Autodesk Inventor part; units mm, degrees
ref_plane "YZ Plane" through (0, 0, 0) normal (1, 0, 0) x (0, 1, 0)
ref_plane "XZ Plane" through (0, 0, 0) normal (0, 1, 0) x (-1, 0, 0)
ref_plane "XY Plane" through (0, 0, 0) normal (0, 0, 1) x (1, 0, 0)
sketch "Sketch1" plane through (0, 0, 0) normal (1, 0, 0) x (0, 1, 0)
  circle A0 centre (0, 0) radius 12.7
  circle A1 centre (0, 0) radius 111.9
  dimension "D_eje" = 25.4
  dimension "d1" = 223.8
extrude "Extrusion1" add sketch "Sketch1" along normal blind 9
sketch "Sketch2" plane through (9, 0, 0) normal (1, 0, 0) x (0, 0, -1)
  line L0 (6, 19.0264) -> (6, 99.7197)
  line L1 (0, -188.1875) -> (0, 173.8632) construction
  arc A0 (0, 19.95) -> (-13.4773, 14.7093) centre (0, 0) ccw construction
  circle A1 centre (0, 0) radius 12.7 construction
  arc A2 (0, 99.9) -> (86.5159, -49.95) centre (0, 0) ccw construction
  line L2 (181.1282, 0) -> (-189.3983, 0) construction
  arc A3 (6, 19.0264) -> (0, 19.95) centre (0, 0) ccw construction
  arc A4 (-19.95, 0) -> (0, -19.95) centre (0, 0) ccw construction
  arc A5 (0, -19.95) -> (17.2772, -9.975) centre (0, 0) ccw construction
  arc A6 (19.95, 0) -> (6, 19.0264) centre (0, 0) ccw
  line L3 (0, 0) -> (86.5159, -49.95) construction
  line L4 (19.4773, -4.317) -> (89.3598, -44.6637)
  arc A7 (-13.4773, 14.7093) -> (-19.95, 0) centre (0, 0) ccw construction
  arc A8 (19.4773, -4.317) -> (19.95, 0) centre (0, 0) ccw
  arc A9 (17.2772, -9.975) -> (19.4773, -4.317) centre (0, 0) ccw construction
  arc A10 (6, 99.7197) -> (0, 99.9) centre (0, 0) ccw construction
  arc A11 (86.5159, -49.95) -> (89.3598, -44.6637) centre (0, 0) ccw construction
  arc A12 (89.3598, -44.6637) -> (6, 99.7197) centre (0, 0) ccw
  line L5 (-19.4773, -4.317) -> (-89.3598, -44.6637)
  arc A13 (-6, 99.7197) -> (-89.3598, -44.6637) centre (0, 0) ccw
  line L6 (-6, 19.0264) -> (-6, 99.7197)
  arc A14 (-9.975, 17.2772) -> (-19.4773, -4.317) centre (0, 0) ccw
  line L7 (13.4773, -14.7093) -> (83.3598, -55.056)
  arc A15 (-83.3598, -55.056) -> (83.3598, -55.056) centre (0, 0) ccw
  line L8 (-13.4773, -14.7093) -> (-83.3598, -55.056)
  arc A16 (-9.975, -17.2772) -> (13.4773, -14.7093) centre (0, 0) ccw
  point P0 (-6, -19.0264)
  point P1 (19.4773, 4.317)
  dimension "d4" = 6
  dimension "d7" = 39.9
  dimension "d8" = 199.8
  dimension "d10" = 120
  dimension "d11" = 6
  dimension "d14" = 360
extrude "Extrusion2" cut sketch "Sketch2" against normal blind 9
pattern_circular "Circular Pattern1" count 3 over 360 about axis through (-10, 0, 0) along (1, 0, 0) of "Extrusion2"
fillet "Fillet1" radius 2 12 edges at (4.5, -14.7093, -13.4773) (4.5, -14.7093, 13.4773) (4.5, -55.056, 83.3598) (4.5, -55.056, -83.3598) (4.5, -44.6637, -89.3598) (4.5, 99.7197, -6) (4.5, -4.317, -19.4773) (4.5, 19.0264, -6) (4.5, 19.0264, 6) (4.5, -4.317, 19.4773) (4.5, 99.7197, 6) (4.5, -44.6637, 89.3598)
properties part number "Rueda_triciclo" material "Aluminum 6061"
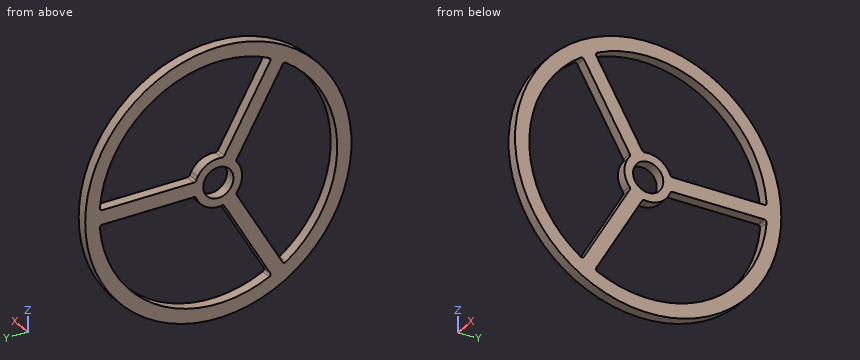
CAD build for the part. Positions are in the model's coordinates, mm. Give positions to 0.01 mm unless a question says otherwise; leave off trailing zeros. Order: outer loops, then holes, each group sorted by start corner. A loop starts at its lowest first (then second) coordinate and runs counter-clockwise, first axis right, second up.
(1) Saw through at C-C, the plane y = 68.5. Give the cut face in (x, z), then the cut area to 3 significant figures.
(2) Saw through at D-D, the plane x = 3.25. State how many separate pieces and enclosed holes the cut face has, then the cut area to 3 significant figures.
(3) Saw through at A-A, the plane z = 0. Give the cut face in (x, y), then the cut area to 3 significant figures.
(4) Drill centre lines: L1, parallel to Z at x = 2, y = 0; L2, parallel to Z at x = 1.5, y = 26.5; L3, parallel to Z at x = 5.75, y = -5.5. Where is each one in solid material? Low to high.
(5) Saw through at B-B, the plane y = -24.5. Give the cut face in (x, z).
(6) Flat gauge pins, fed straight in: pin 1 (1.5 mm diameter, centred on x = 6, z = 69.5, fed in from +Y); pin 2 (2 mm diameter, centred on x = 2.5, y = -34.5, fed in from -Z); pin 3 (4.5 mm diameter, centred on x = 4.5, y = 40.5, fed in from +Z); pin 4 (4 mm diameter, centred on y = 46, z = 88, fed in from -X). Where does each tip first touch, or does it go through?
Results found:
1. outline: (0, -88.48) - (9, -88.48) - (9, -72.72) - (0, -72.72) - close; (0, -6) - (9, -6) - (9, 6) - (0, 6) - close; (0, 72.72) - (9, 72.72) - (9, 88.48) - (0, 88.48) - close
1. area: 392 mm2
2. separate pieces: 1
2. enclosed holes: 4
2. area: 11,600 mm2
3. outline: (0, -111.9) - (9, -111.9) - (9, -99.9) - (0, -99.9) - close; (0, -19.95) - (9, -19.95) - (9, -12.7) - (0, -12.7) - close; (0, 12.7) - (9, 12.7) - (9, 111.9) - (0, 111.9) - close
3. area: 1,070 mm2
4. L1: z = -111.9 to -99.9, -19.95 to -12.7, 12.7 to 19.95, 99.9 to 111.9
4. L2: z = -108.72 to -96.32, -6 to 6, 96.32 to 108.72
4. L3: z = -111.76 to -99.75, -21.53 to -11.45, 11.45 to 21.53, 99.75 to 111.76
5. outline: (0, -109.18) - (9, -109.18) - (9, -96.85) - (0, -96.85) - close; (0, -54.44) - (9, -54.44) - (9, -30.44) - (0, -30.44) - close; (0, 30.44) - (9, 30.44) - (9, 54.44) - (0, 54.44) - close; (0, 96.85) - (9, 96.85) - (9, 109.18) - (0, 109.18) - close
6. pin 1: stops at y = 88.29
6. pin 2: stops at z = -106.77
6. pin 3: stops at z = 105.16
6. pin 4: stops at x = 0
